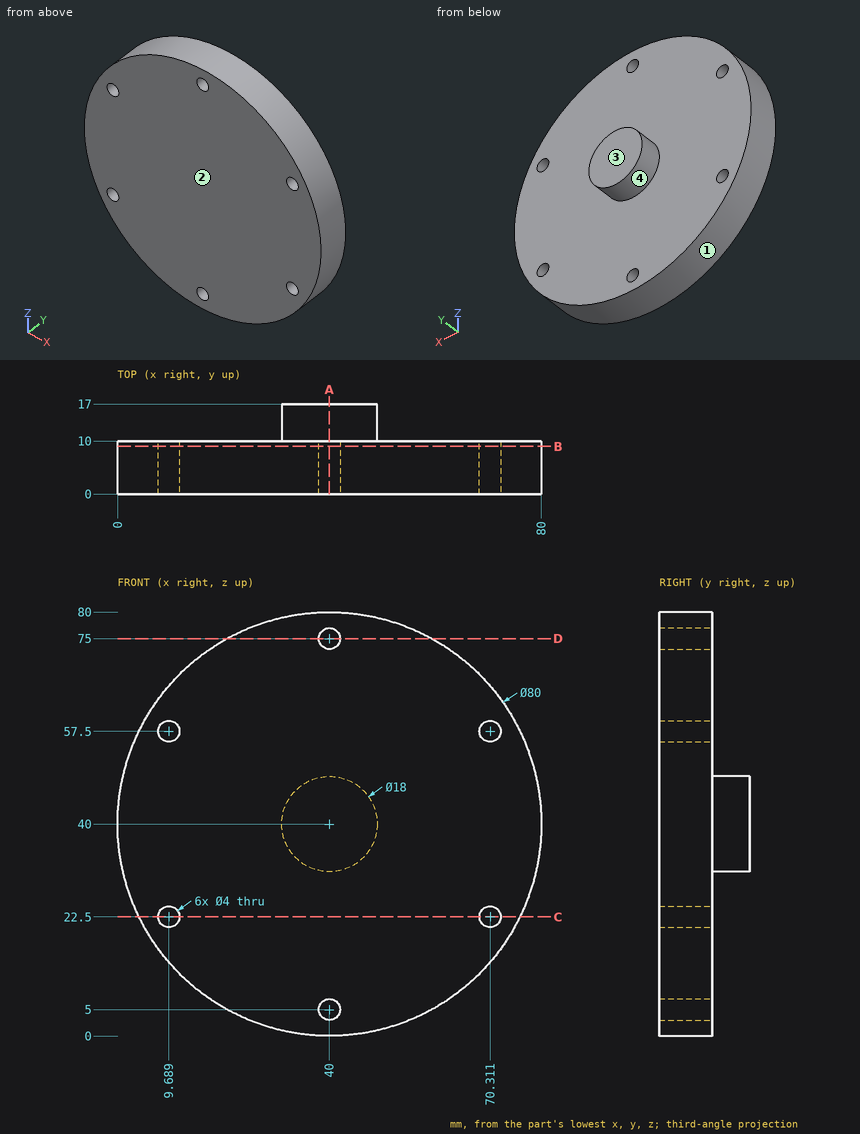
Part print with two shaded views. Sizes in mm from the minimum x, y, z corner. A direction names the side the tool comes from. Round coordinates to 2 decimals unless told otherwise and drop trailing zeros. Loops run counter-clockwise (first coordinate to the right, second up) from the corner with the lowest first, then second, coordinate; pieces in that order, holes last. Notation, with made-up numbers: M 69.5,24.5 L 99.5,24.5 A18 cw 99.5,34.5 Z; hole C 14,32.25 d6. An arc over 180 degrees is marked long. Put each result on its own line as item: value. Start each with the question number.
Item 1: Cut at A-A (x = 40). List the corners of the cut face in (y, z), then the cut area to 3 significant figures.
Item 2: Drop flat-ended pins along their axis: P1, Ø10, axis at x = 56, z = 27.5, coming from the +Y side; P2, Ø3, axis at x = 56.5, y = 7, coming from the +Z side; P3, Ø2, axis at x = 41.5, y = 13.5, coming from the +Z side. Give the stop position or say it passes through.
Item 3: Cut at D-D (z = 75). List the corners of the cut face in (x, y) (3 decimals), then the cut area to 3 significant figures.
Item 4: Drill centre lines: line 1 along Z through (x, y) = (40, 3); line 2 along X through (y, z) = (5, 22.5); line 3 along Z through (x, y) = (40.5, 7.25). Where is each one in solid material? Low to high.
Item 5: Cut at B-B (y = 9). List the corners of the cut face in (x, z).
Item 6: Mould opens along X. For the marked faces 1 and 2 say: released by +X, released by -X, zero draft, split by the parting line, or undercut.
Item 7: Cut at C-C (z = 22.5). List the corners of the cut face in (x, y), then the cut area to 3 significant figures.
Item 8: 3-axis set-ups, long thin cutter, end or side, ignore diameter. For the marked faces 3 and 4: which of +Z, -Z, +X, -X, +Y, -Y reach the whole face in a straight line?
Answer block:
1. outline: M 0,0 L 10,0 L 10,3 L 0,3 Z; M 0,7 L 10,7 L 10,31 L 17,31 L 17,49 L 10,49 L 10,73 L 0,73 Z; M 0,77 L 10,77 L 10,80 L 0,80 Z
1. area: 846 mm2
2. P1: y = 10
2. P2: z = 77.08
2. P3: z = 48.99
3. outline: M 20.635,0 L 38,0 L 38,10 L 20.635,10 Z; M 42,0 L 59.365,0 L 59.365,10 L 42,10 Z
3. area: 347 mm2
4. line 1: 0 to 3, 7 to 73, 77 to 80
4. line 2: 4.03 to 7.69, 11.69 to 68.31, 72.31 to 75.97
4. line 3: 0 to 3.06, 6.94 to 73.06, 76.94 to 80
5. outline: C 40,40 d80; hole C 9.69,22.5 d4; hole C 9.69,57.5 d4; hole C 40,5 d4; hole C 40,75 d4; hole C 70.31,22.5 d4; hole C 70.31,57.5 d4
6. face 1: split by the parting line
6. face 2: zero draft
7. outline: M 4.03,0 L 7.69,0 L 7.69,10 L 4.03,10 Z; M 11.69,0 L 68.31,0 L 68.31,10 L 11.69,10 Z; M 72.31,0 L 75.97,0 L 75.97,10 L 72.31,10 Z
7. area: 639 mm2
8. face 3: +Z, -Z, +X, -X, +Y
8. face 4: +Y
